Can you work these out from the model? Positions are in its coordinate system, mm. Face numbers are marked on the shaded views. A direction names the side the tool comes from. Round coordinates to 2 decimals unless told otherwise and drop trailing zeros. Loops run counter-clockwise (first coordinate to the right, second up) from the corner with the lowest first, then second, coordinate; pieces in that order, holes last. Notation, with made-up numbers: M -3.75,63.25 L 26.25,63.25 A26 cw 26.25,88.25 Z; hole C 84,-25.5 d3. An arc over 180 degrees is marked long. Answer as CSV lines item,"result".
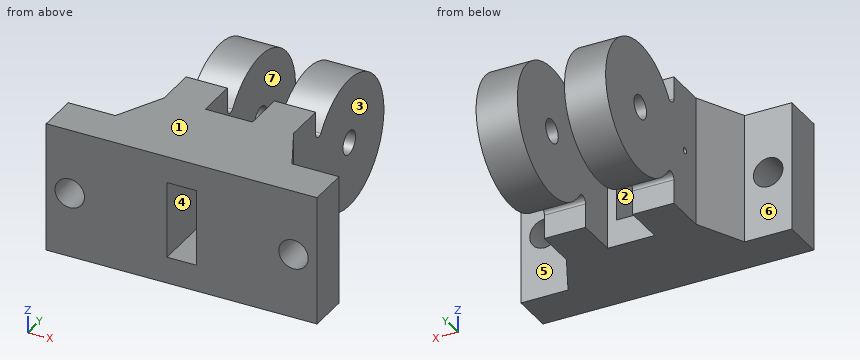
from build123d import *

# Parameters (mm, degrees)
SKETCH1_W                      = 22
SKETCH1_H                      = 22
BODY_BASE_DEPTH                = 20
SKETCH8_W                      = 22
SKETCH8_H                      = 5
CHANNEL_FOR_TENDONS_DEPTH      = 4
BOSS_EXTRUDE2_DEPTH            = 7
LPATTERN1_COUNT                = 2
LPATTERN1_PITCH                = 15
SKETCH11_R                     = 2
CONNECT_TO_GRIPPERS_DEPTH      = 23
BOSS_EXTRUDE3_DEPTH            = 11
SKETCH13_R                     = 2.5
CUT_EXTRUDE3_DEPTH             = 8
SKETCH16_W                     = 5
SKETCH16_H                     = 13
TENDON_PASS_THROUGH_HOLE_DEPTH = 16
SKETCH17_R                     = 0.5
TENDON_PIN_HOLE_DEPTH          = 35


with BuildPart() as part:
    # Sketch1 → Body Base (new body)
    with BuildSketch(Plane(origin=(0, 0, 0), x_dir=(1, 0, 0), z_dir=(0, 1, 0))):
        Rectangle(SKETCH1_W, SKETCH1_H)
    extrude(amount=BODY_BASE_DEPTH)

    # Sketch8 → Channel for Tendons (cut, symmetric)
    with BuildSketch(Plane(origin=(0, 0, 0), x_dir=(0, 0, -1), z_dir=(1, 0, 0))):
        with Locations((0, 17.5)):
            Rectangle(SKETCH8_W, SKETCH8_H)
    extrude(amount=CHANNEL_FOR_TENDONS_DEPTH, both=True, mode=Mode.SUBTRACT)

    # Sketch9 → Boss-Extrude2 (add)
    with BuildSketch(Plane(origin=(11, 0, 0), x_dir=(0, 0, -1), z_dir=(1, 0, 0))):
        with BuildLine():
            Line((-11, 20), (-11, 22))
            Line((-11, 22), (-7.188338132, 22))
            ThreePointArc((-7.188338132, 22), (-6.278997638, 22.58394728), (-6.43167096, 23.653800269))
            ThreePointArc((-6.43167096, 23.653800269), (-0.13450677, 43.67298666), (6.16265742, 23.653800269))
            ThreePointArc((6.16265742, 23.653800269), (6.009984097, 22.58394728), (6.919324592, 22))
            Line((6.919324592, 22), (11, 22))
            Line((11, 22), (11, 20))
            Line((11, 20), (-11, 20))
        make_face()
    boss_extrude2 = extrude(amount=-BOSS_EXTRUDE2_DEPTH)

    # LPattern1: Boss-Extrude2 ×2
    with Locations(*[(-i * LPATTERN1_PITCH, 0, 0) for i in range(1, LPATTERN1_COUNT)]):
        add(boss_extrude2)

    # Sketch11 → Connect to Grippers (cut, through all)
    with BuildSketch(Plane(origin=(11, 0, 0), x_dir=(0, 0, -1), z_dir=(1, 0, 0))):
        with Locations((-0.13450677, 32.67298666)):
            Circle(SKETCH11_R)
    extrude(amount=-CONNECT_TO_GRIPPERS_DEPTH, mode=Mode.SUBTRACT)

    # Sketch12 → Boss-Extrude3 (add, symmetric)
    with BuildSketch(Plane.XY):
        Polygon((-11, 15), (-15, 7), (-23, 7), (-23, 0), (-11, 0), align=None)
        Polygon((11, 15), (15, 7), (23, 7), (23, 0), (11, 0), align=None)
    extrude(amount=BOSS_EXTRUDE3_DEPTH, both=True)

    # Sketch13 → Cut-Extrude3 (cut, through all)
    with BuildSketch(Plane(origin=(0, 7, 0), x_dir=(1, 0, 0), z_dir=(0, 1, 0))):
        with Locations((-19, 0)):
            Circle(SKETCH13_R)
        with Locations((19, 0)):
            Circle(SKETCH13_R)
    extrude(amount=-CUT_EXTRUDE3_DEPTH, mode=Mode.SUBTRACT)

    # Sketch16 → Tendon Pass Through Hole (cut, through all)
    with BuildSketch(Plane(origin=(0, 15, 0), x_dir=(1, 0, 0), z_dir=(0, 1, 0))):
        Rectangle(SKETCH16_W, SKETCH16_H)
    extrude(amount=-TENDON_PASS_THROUGH_HOLE_DEPTH, mode=Mode.SUBTRACT)

    # Sketch17 → Tendon Pin Hole (cut, through all)
    with BuildSketch(Plane.ZY.offset(11)):
        with Locations((0, 18.5)):
            Circle(SKETCH17_R)
    extrude(amount=-TENDON_PIN_HOLE_DEPTH, mode=Mode.SUBTRACT)


solid = part.part
Item 1: If we section it at C-C on z = -8.75: Write out the boundary of the cut face in (x, y), then the cut area to 3 significant figures.
Output:
outline,"M -23,0 L 23,0 L 23,7 L 15,7 L 11,15 L 11,22 L 4,22 L 4,15 L -4,15 L -4,22 L -11,22 L -11,15 L -15,7 L -23,7 Z; M -11,26.19 L -4,26.19 L -4,39.16 L -11,39.16 Z; M 4,26.19 L 11,26.19 L 11,39.16 L 4,39.16 Z"
area,"810 mm2"
Item 2: If we section it at A-A on x = 19: Write out the boundary of the cut face in (y, z), then the cut area to 3 significant figures.
Output:
outline,"M 0,-11 L 7,-11 L 7,-2.5 L 0,-2.5 Z; M 0,2.5 L 7,2.5 L 7,11 L 0,11 Z"
area,"119 mm2"
Item 3: Will these pins go through, and if not, where does the flat tip stop? pin 1 (6 mm diameter, centred on x = 19, z = 0, fed in from +Y); pin 2 (10 mm diameter, centred on y = 19, z = -5.5, fed in from -X); pin 3 (24 mm diameter, centred on x = 11, y = 13, fed in from +Z); pin 4 (2.5 mm diameter, centred on x = -1, z = -2.5, fed in from +Y).
Output:
pin 1,"stops at y = 7"
pin 2,"stops at x = -11.5"
pin 3,"stops at z = 11"
pin 4,"passes through"
Item 4: If we section it at B-B on y = 10.5: Write out the boundary of the cut face in (x, z).
Output:
outline,"M -13.25,-11 L 13.25,-11 L 13.25,11 L -13.25,11 Z; hole M -2.5,-6.5 L 2.5,-6.5 L 2.5,6.5 L -2.5,6.5 Z"
Item 5: If we section it at D-D on y = 6: Write out the boundary of the cut face in (x, z).
Output:
outline,"M -23,-11 L 23,-11 L 23,11 L -23,11 Z; hole C -19,0 d5; hole M -2.5,-6.5 L 2.5,-6.5 L 2.5,6.5 L -2.5,6.5 Z; hole C 19,0 d5"
Item 6: We'd pull the mould along Z, two halves only. Please class the marked faces 1, 2 and 3: released by +Z, released by -Z, zero draft, split by the parting line, or undercut.
Output:
face 1,"released by +Z"
face 2,"undercut"
face 3,"zero draft"
Item 7: On a 3-axis mill with a long thin cutter (end or side, diameter ignored), from which of +Z, -Z, +X, -X, +Y, -Y can I reach the whole of each face in a straight line? I mean the marked faces 4, 5, 6 and 7. Say none if no direction works.
Output:
face 4,"+Y, -Y"
face 5,"+Z, -Z, +X, +Y"
face 6,"+Z, -Z, -X, +Y"
face 7,"+Z, -Z, +Y"
Item 8: If I drill on line 1 along X through (y, z) = (3.25, 0); line 2 along Y through (x, z) = (-7, 0); line 3 along Z through (x, y) = (19, 2.75), over which ranges is the centre line in solid material (lowest first)? Write a range as from..to.
Output:
line 1,"x = -23..-21.5, -16.5..-2.5, 2.5..16.5, 21.5..23"
line 2,"y = 0..18, 19..30.68, 34.67..43.67"
line 3,"z = -11..-2.5, 2.5..11"
